Here's the drawing with two shaded views (mm, measured from the low corner). I have some questions. A direction names the side the tool comes from. Round coordinates to 2 decimals unless told otherwise and drop trailing zeros. Loops run counter-clockwise (first coordinate to the right, second up) from the corner with the lowest first, then second, coordinate; pieces in that order, holes last.
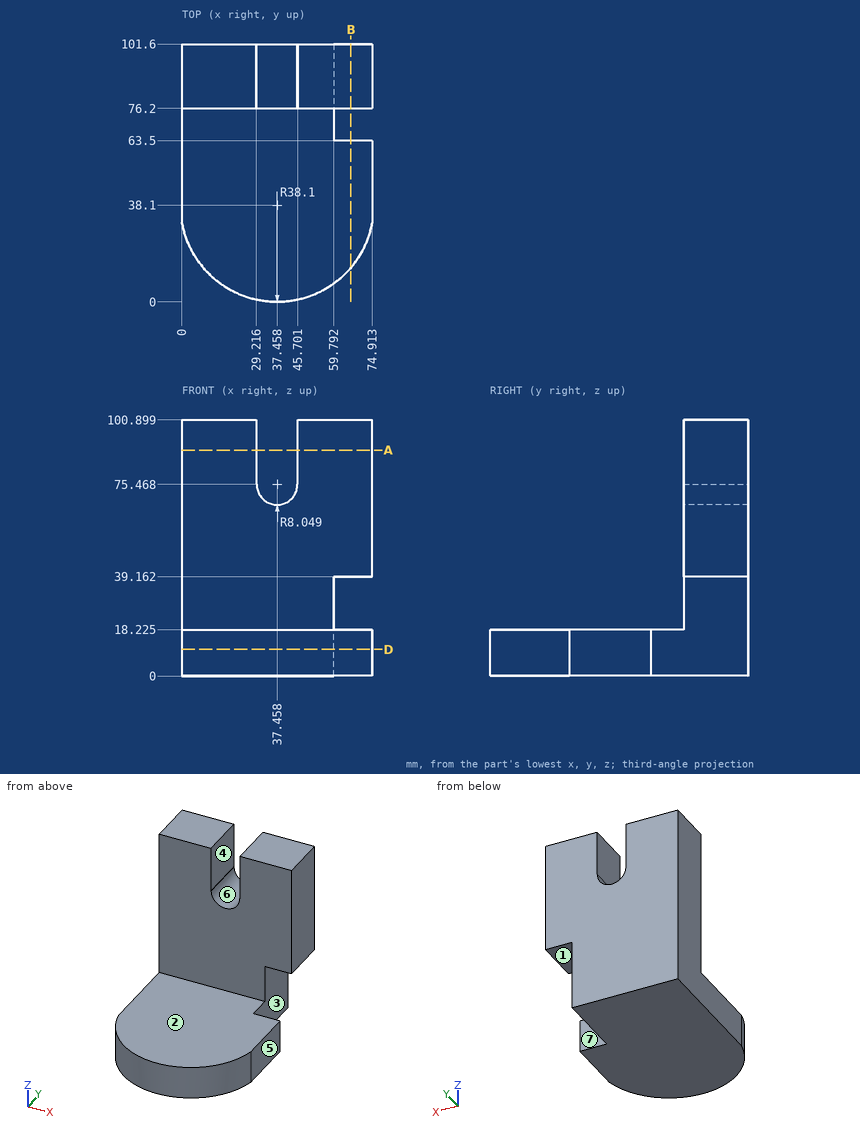
Item 1: If I drill on line 1 along Z through (x, y) = (64.5, 63) (1 decimal); line 2 along Y through (x, z) = (25.5, 73); line 3 along Z through (x, y) = (64, 93.5), over which ranges is the centre line in solid material (lowest first)?
Results list:
line 1: z = 0 to 18.2
line 2: y = 76.2 to 101.6
line 3: z = 39.16 to 100.9
Item 2: If we section it at A-A, the plane z = 89: Please give me the cut outline in (x, y) (1 decimal), then the cut area to 3 significant figures.
Results list:
outline: (0, 76.2) - (29.2, 76.2) - (29.2, 101.6) - (0, 101.6) - close; (45.7, 76.2) - (74.9, 76.2) - (74.9, 101.6) - (45.7, 101.6) - close
area: 1,480 mm2
Item 3: We'd pull the mould along X, two halves only. Please class the marked faces 5, 6 and 7: released by +X, released by -X, zero draft, split by the parting line, or undercut.
Results list:
face 5: released by +X
face 6: undercut
face 7: zero draft
Item 4: Will these pins go through, and if not, where does the flat tip stop? pin 1 (3 mm diameter, centred on x = 51.5, y = 39, fed in from +Z) (1 decimal); pin 2 (7.5 mm diameter, centred on x = 65.5, y = 85.5, fed in from -Z); pin 3 (22.5 mm diameter, centred on x = 49.5, z = 64.5, fed in from -Y).
Results list:
pin 1: stops at z = 18.2
pin 2: stops at z = 39.16
pin 3: stops at y = 76.2
Item 5: If we section it at D-D, the plane z = 10.5: Please give me the cut outline in (x, y).
Results list:
outline: (0, 31.14) arc R38.1 ccw to (74.91, 31.12) - (74.91, 63.5) - (59.79, 63.5) - (59.79, 101.6) - (0, 101.6) - close
Item 6: If we section it at B-B, the plane x = 66.5: Please give me the cut outline in (y, z) (1 decimal).
Results list:
outline: (13.4, 0) - (63.5, 0) - (63.5, 18.2) - (13.4, 18.2) - close; (76.2, 39.2) - (101.6, 39.2) - (101.6, 100.9) - (76.2, 100.9) - close
Item 7: For the marked faces 1, 2, 3 and 4, which set-ups out of +Z, -Z, +X, -X, +Y, -Y let a thin tool reach every point of the face, with its end or its side?
Results list:
face 1: -Z, +X, +Y, -Y
face 2: +Z, +X, -X, -Y
face 3: -Z, +X, +Y
face 4: +Z, +Y, -Y
